Could you check a few things on this model? Use its own coordinates, in mm. A direction names the side the tool comes from. Coordinates: 2 decimals unless noted, no trailing zeros. Order: outer loops, then holes, each group sorted by start corner. A loop starts at its lowest first (then second) coordinate and runs counter-clockwise, first axis right, second up. Notation, with made-up numbers: (82, 87.25) - (86, 87.25) arc R22 cw to (86, 110.25) - close; hole circle Ø11 at (28, -17). An arc over 180 degrees is marked (long way). Answer as CSV lines item,"result". Start each with the question number.
1. I want a section at D-D, the plane y = 33. List the corners of the cut face in (x, z) for me.
2. I need wall thicknesses on probe 1 along Y at (x, z) = (50.25, 1) (3 decimals); probe 2 along Y at (x, z) = (3.5, 2.5); probe 3 along X at (y, z) = (26, 8.5). Which ranges of each line are inside material? Lowest first, please.
3. I want a section at B-B, the plane x = 47.45. List the corners of the cut face in (y, z) for me, and give its area (3 significant figures).
4. For faces 1 (the face through (38.123, 42, 4)), 2 (the face through (-0.3, 20, 4)), 3 (the face through (52, 32, 6.5)), which set-ups out of +Z, -Z, +X, -X, +Y, -Y let a thin tool reach every point of the face, with its end or its side?
5. Thinking about a two-plate mould opening in Z: for faces 4 (the face through (16, 42, 6.5)), 5 (the face through (24, 41.68, 1)), 6 (the face through (24.3, 20.4, -4.5)), which applies, released by +Z, released by -Z, zero draft, split by the parting line, or undercut?
6. I want a section at C-C, the plane x = 19. List the corners of the cut face in (y, z) for me, and give its area (3 significant figures).
7. For pin 1 (1 mm diameter, centred on x = 18.5, y = 5, fed in from +Z); pin 2 (2 mm diameter, centred on x = 47.45, y = 39.357, fed in from +Z), each with a flat end and sliding along its axis, tell me the tip position at first contact or that it passes through.
8. I want a section at A-A, the plane y = 2. List the corners of the cut face in (x, z) for me, and give its area (3 significant figures).
from build123d import *
from build123d.topology import SkipClean

# Parameters (mm, degrees)
EXTRUDE_START             = -4.5
SKETCH_3_W                = 52.75
SKETCH_3_H                = 44.78
EXTRUDE_1_DEPTH           = 2
HOLE_WIZARD_M2_1_D        = 1.6
CUT_EXTRUDE_START         = -2.5
SKETCH_3_5_W              = 9.2
SKETCH_3_5_H              = 7.5
SKETCH_3_5_W_2            = 7.5
SKETCH_3_5_H_2            = 9.2
CUT_EXTRUDE_2_DEPTH       = 0.5
SKETCH_3_6_W              = 52.75
SKETCH_3_6_H              = 44.78
SKETCH_3_6_W_2            = 49.95
SKETCH_3_6_H_2            = 41.98
EXTRUDE_3_DEPTH           = 15.6
SKETCH_10_R               = 1
CUT_EXTRUDE_5_DEPTH       = 70.004774472
SKETCH_13_W               = 4.5
SKETCH_13_H               = 9.2
CUT_EXTRUDE_6_DEPTH       = 2
SKETCH_14_W               = 9.2
SKETCH_14_H               = 4.5
SKETCH_14_W_2             = 21
CUT_EXTRUDE_7_DEPTH       = 2
SKETCH_15_W               = 4.5
SKETCH_15_H               = 7.5
CUT_EXTRUDE_8_DEPTH       = 2
M1_2X0_25_2_D             = 0.95
PCB_4_5_3_M2_1_6_START    = -2.5
SKETCH_23_R               = 1.5
SKETCH_23_R_2             = 0.8
PCB_4_5_3_M2_1_6_DEPTH    = 4.5
SKETCH_26_W               = 15.6
SKETCH_26_H               = 44.78
EXTRUDE_2_6_4_DEPTH       = 2.6
SKETCH_27_W               = 15.6
SKETCH_27_H               = 44.78
EXTRUDE_2_6_4_2_DEPTH     = 2.6
SKETCH_28_R               = 1.3
SKETCH_28_R_2             = 2.05
SKETCH_28_W               = 4.5
SKETCH_28_H               = 7.5
SMA_4X2_6_4_1_USB_DEPTH   = 4
SMA_4X2_6_4_1_USB_START   = -4
SKETCH_29_R               = 1.3
SKETCH_29_R_2             = 2.05
SKETCH_29_W               = 4.5
SKETCH_29_H               = 9.2
SMA_4X2_6_4_1_USB_2_DEPTH = 4


with BuildPart() as part:
    # 草图3 → 凸台-拉伸1 (new body)
    with BuildSketch(Plane.XY.offset(EXTRUDE_START)):
        with Locations((24.675, 20.69)):
            Rectangle(SKETCH_3_W, SKETCH_3_H)
    extrude(amount=EXTRUDE_1_DEPTH)

    # M2 螺纹孔1 (through all)
    with Locations(Plane(origin=(2.003, 2, -2.5), x_dir=(1, 0, 0), z_dir=(0, 0, 1))):
        with Locations((0, 0), (45.447, 0), (45.447, 37.357), (0, 37.357), (21.222, 18.3)):
            Hole(HOLE_WIZARD_M2_1_D / 2)

    # 草图3<5> → 切除-拉伸2 (cut)
    with BuildSketch(Plane.XY.offset(CUT_EXTRUDE_START)):
        with Locations((33.523, 37.63)):
            Rectangle(SKETCH_3_5_W, SKETCH_3_5_H)
        with Locations((45.6, 31.7)):
            Rectangle(SKETCH_3_5_W_2, SKETCH_3_5_H_2)
    extrude(amount=-CUT_EXTRUDE_2_DEPTH, mode=Mode.SUBTRACT)

    # 草图3<6> → 凸台-拉伸3 (add)
    with BuildSketch(Plane.XY.offset(EXTRUDE_START)):
        with Locations((24.675, 20.69)):
            Rectangle(SKETCH_3_6_W, SKETCH_3_6_H)
        with Locations((24.675, 20.69)):
            Rectangle(SKETCH_3_6_W_2, SKETCH_3_6_H_2, mode=Mode.SUBTRACT)
    extrude(amount=EXTRUDE_3_DEPTH)

    # 草图10 → 切除-拉伸5 (cut, through all)
    with BuildSketch(Plane.ZY.offset(1.7)):
        with Locations((3.3, 10.725)):
            Circle(SKETCH_10_R)
    extrude(amount=-CUT_EXTRUDE_5_DEPTH, mode=Mode.SUBTRACT)

    # 草图13 → 切除-拉伸6 (cut)
    with BuildSketch(Plane(origin=(51.05, 0, 0), x_dir=(0, 0, -1), z_dir=(1, 0, 0))):
        with Locations((-4.25, 31.65)):
            Rectangle(SKETCH_13_W, SKETCH_13_H)
    extrude(amount=-CUT_EXTRUDE_6_DEPTH, mode=Mode.SUBTRACT)

    # 草图14 → 切除-拉伸7 (cut)
    with BuildSketch(Plane(origin=(0, 43.08, 0), x_dir=(1, 0, 0), z_dir=(0, 1, 0))):
        with Locations((33.523, -4.25)):
            Rectangle(SKETCH_14_W, SKETCH_14_H)
        with Locations((16.57, -4.25)):
            Rectangle(SKETCH_14_W_2, SKETCH_14_H)
    extrude(amount=-CUT_EXTRUDE_7_DEPTH, mode=Mode.SUBTRACT)

    # 草图15 → 切除-拉伸8 (cut)
    with BuildSketch(Plane.ZY.offset(1.7)):
        with Locations((4.25, 30.2)):
            Rectangle(SKETCH_15_W, SKETCH_15_H)
    extrude(amount=-CUT_EXTRUDE_8_DEPTH, mode=Mode.SUBTRACT)

    # M1.2x0.25 螺纹孔2 (through all)
    with Locations(Plane(origin=(-0.8, -0.8, 11.1), x_dir=(1, 0, 0), z_dir=(0, 0, 1))):
        with Locations((0, 0), (51.05, 0), (51.05, 43.08), (0, 43.08)):
            Hole(M1_2X0_25_2_D / 2)

    # 草图23 → 保持PCB原高度的五处支撑柱_高4.5_外径3_M2底孔1.6 (add)
    # profile 1 of 5: a face of its own
    with SkipClean():  # the faces are left unmerged after this step: merging them gives an invalid solid
        with BuildSketch(Plane.XY.offset(PCB_4_5_3_M2_1_6_START)):
            with Locations(Location((23.225, 20.3, 0), (0, 0, 180))):
                Circle(SKETCH_23_R)
            with Locations((23.225, 20.3)):
                Circle(SKETCH_23_R_2, mode=Mode.SUBTRACT)
        # profile 2 of 5: a face of its own
        with BuildSketch(Plane.XY.offset(PCB_4_5_3_M2_1_6_START)):
            with Locations(Location((2.003, 39.357, 0), (0, 0, 180))):
                Circle(SKETCH_23_R)
            with Locations((2.003, 39.357)):
                Circle(SKETCH_23_R_2, mode=Mode.SUBTRACT)
        # profile 3 of 5: a face of its own
        with BuildSketch(Plane.XY.offset(PCB_4_5_3_M2_1_6_START)):
            with Locations(Location((47.45, 39.357, 0), (0, 0, 180))):
                Circle(SKETCH_23_R)
            with Locations((47.45, 39.357)):
                Circle(SKETCH_23_R_2, mode=Mode.SUBTRACT)
        # profile 4 of 5: a face of its own
        with BuildSketch(Plane.XY.offset(PCB_4_5_3_M2_1_6_START)):
            with Locations(Location((47.45, 2, 0), (0, 0, 180))):
                Circle(SKETCH_23_R)
            with Locations((47.45, 2)):
                Circle(SKETCH_23_R_2, mode=Mode.SUBTRACT)
        # profile 5 of 5: a face of its own
        with BuildSketch(Plane.XY.offset(PCB_4_5_3_M2_1_6_START)):
            with Locations(Location((2.003, 2, 0), (0, 0, 180))):
                Circle(SKETCH_23_R)
            with Locations((2.003, 2)):
                Circle(SKETCH_23_R_2, mode=Mode.SUBTRACT)
        extrude(amount=PCB_4_5_3_M2_1_6_DEPTH)
    add(part.part.scale(1), mode=Mode.REPLACE)  # the faces are merged on a copy

    # 草图26 → Extrude 2.6__4 (add)
    with BuildSketch(Plane.ZY.offset(1.7)):
        with Locations((3.3, 20.69)):
            Rectangle(SKETCH_26_W, SKETCH_26_H)
    extrude(amount=EXTRUDE_2_6_4_DEPTH)

    # 草图27 → Extrude 2.6__4 2 (add)
    with BuildSketch(Plane(origin=(51.05, 0, 0), x_dir=(0, 0, -1), z_dir=(1, 0, 0))):
        with Locations((-3.3, 20.69)):
            Rectangle(SKETCH_27_W, SKETCH_27_H)
    extrude(amount=EXTRUDE_2_6_4_2_DEPTH)

    # 草图28 → SMA__4x2.6__4.1__USB (cut)
    with BuildSketch(Plane.ZY.offset(4.3)):
        with Locations((-0.400503673, 6.425)):
            Circle(SKETCH_28_R)
        with Locations((8.199496327, 6.425)):
            Circle(SKETCH_28_R)
        with Locations((-0.400503673, 15.025)):
            Circle(SKETCH_28_R)
        with Locations((8.199496327, 15.025)):
            Circle(SKETCH_28_R)
        with Locations((3.899496327, 10.725)):
            Circle(SKETCH_28_R_2)
        with Locations((4.25, 30.2)):
            Rectangle(SKETCH_28_W, SKETCH_28_H)
    extrude(amount=-SMA_4X2_6_4_1_USB_DEPTH, mode=Mode.SUBTRACT)

    # 草图29 → SMA__4x2.6__4.1__USB 2 (cut)
    with SkipClean():  # the faces are left unmerged after this step: merging them gives an invalid solid
        with BuildSketch(Plane(origin=(53.65, 0, 0), x_dir=(0, 0, -1), z_dir=(1, 0, 0)).offset(SMA_4X2_6_4_1_USB_START)):
            with Locations(Location((0.400503673, 6.425, 0), (0, 0, 180))):
                Circle(SKETCH_29_R)
            with Locations(Location((-8.199496327, 6.425, 0), (0, 0, 180))):
                Circle(SKETCH_29_R)
            with Locations(Location((0.400503673, 15.025, 0), (0, 0, 180))):
                Circle(SKETCH_29_R)
            with Locations(Location((-8.199496327, 15.025, 0), (0, 0, 180))):
                Circle(SKETCH_29_R)
            with Locations(Location((-3.899496327, 10.725, 0), (0, 0, 180))):
                Circle(SKETCH_29_R_2)
            with Locations((-4.25, 31.65)):
                Rectangle(SKETCH_29_W, SKETCH_29_H)
        extrude(amount=SMA_4X2_6_4_1_USB_2_DEPTH, mode=Mode.SUBTRACT)


solid = part.part
Solved:
1,outline,"(-4.3, -4.5) - (53.65, -4.5) - (53.65, 2) - (49.65, 2) - (49.65, -2.5) - (49.35, -2.5) - (49.35, -3) - (41.85, -3) - (41.85, -2.5) - (-0.3, -2.5) - (-0.3, 2) - (-4.3, 2) - close; (-4.3, 6.5) - (-0.3, 6.5) - (-0.3, 11.1) - (-4.3, 11.1) - close; (49.65, 6.5) - (53.65, 6.5) - (53.65, 11.1) - (49.65, 11.1) - close"
2,probe 1,"y = -1.7 to -1.275, -0.325 to 41.805, 42.755 to 43.08"
2,probe 2,"y = -1.7 to -0.3, 41.68 to 43.08"
2,probe 3,"x = -4.3 to -0.3, 49.65 to 53.65"
3,outline,"(-1.7, -4.5) - (1.2, -4.5) - (1.2, 2) - (0.5, 2) - (0.5, -2.5) - (-0.3, -2.5) - (-0.3, 11.1) - (-1.7, 11.1) - close; (2.8, -4.5) - (38.56, -4.5) - (38.56, 2) - (37.86, 2) - (37.86, -2.5) - (36.3, -2.5) - (36.3, -3) - (27.1, -3) - (27.1, -2.5) - (3.5, -2.5) - (3.5, 2) - (2.8, 2) - close; (40.16, -4.5) - (43.08, -4.5) - (43.08, 11.1) - (41.68, 11.1) - (41.68, -2.5) - (40.86, -2.5) - (40.86, 2) - (40.16, 2) - close"
3,area,"129 mm2"
4,face 1,"+Y"
4,face 2,"+Z"
4,face 3,"+X"
5,face 4,"undercut"
5,face 5,"zero draft"
5,face 6,"released by -Z"
6,outline,"(-1.7, -4.5) - (43.08, -4.5) - (43.08, 2) - (41.68, 2) - (41.68, -2.5) - (-0.3, -2.5) - (-0.3, 11.1) - (-1.7, 11.1) - close; (41.68, 6.5) - (43.08, 6.5) - (43.08, 11.1) - (41.68, 11.1) - close"
6,area,"121 mm2"
7,pin 1,"stops at z = -2.5"
7,pin 2,"stops at z = 2"
8,outline,"(-4.3, -4.5) - (1.2, -4.5) - (1.2, 2) - (0.5, 2) - (0.5, -2.5) - (-0.3, -2.5) - (-0.3, 11.1) - (-4.3, 11.1) - close; (2.8, -4.5) - (46.65, -4.5) - (46.65, 2) - (45.95, 2) - (45.95, -2.5) - (3.5, -2.5) - (3.5, 2) - (2.8, 2) - close; (48.25, -4.5) - (53.65, -4.5) - (53.65, 11.1) - (49.65, 11.1) - (49.65, -2.5) - (48.95, -2.5) - (48.95, 2) - (48.25, 2) - close"
8,area,"231 mm2"
